Work out the finished part from the listing and answer in its coordinate system (mm). A direction names the side the tool comes from. Round coordinates to 2 decimals unless told otherwise and drop trailing zeros. Write each loop counter-clockwise with the first axis right and the second up, starting at its lowest first coordinate (ties: lowest second). Pieces come first, ordered by that corner, then holes. Notation, with made-up numbers: (-25, 48) -> (31, 48) arc R11 cw to (31, 68) -> close; hole circle Ø8 at (-13, -3). An arc over 180 degrees is marked (long way). One line per question, with ' | ' between items. Start each with the question number.
```python
from build123d import *

# Parameters (mm, degrees)
SKETCH1_R               = 23.8125
BOSS_EXTRUDE1_DEPTH     = 6.35
CUT_EXTRUDE1_DEPTH      = 53.964614985
CUT_EXTRUDE1_DEPTH_BACK = 53.964614985
SKETCH4_R               = 1.75768
BOSS_EXTRUDE3_START     = -6.35
BOSS_EXTRUDE3_DEPTH     = 6.35
SKETCH13_W              = 24.51582
SKETCH13_H              = 34.16660521
BOSS_EXTRUDE7_DEPTH     = 2.2225
SKETCH14_W              = 18.4
SKETCH14_H              = 4.571
BOSS_EXTRUDE8_DEPTH     = 12.423266239
SKETCH19_W              = 1.60782
SKETCH19_H              = 34.16660521
BOSS_EXTRUDE14_DEPTH    = 12.423266239
SKETCH20_W              = 14.645766239
SKETCH20_H              = 34.16660521
BOSS_EXTRUDE15_DEPTH    = 0.455043
CUT_EXTRUDE2_DEPTH      = 4.8895
SKETCH25_W              = 11.467193476
SKETCH25_H              = 6.35
CUT_EXTRUDE3_DEPTH      = 4.7625
SKETCH23_R              = 1.0414
CUT_EXTRUDE4_DEPTH      = 17.78
SKETCH27_R              = 1.0414
CUT_EXTRUDE5_DEPTH      = 12.7
BOSS_EXTRUDE17_START    = -34.16660521
BOSS_EXTRUDE17_DEPTH    = 34.16660521
SKETCH31_W              = 6.35
SKETCH31_H              = 8.89
CUT_EXTRUDE6_DEPTH      = 7.874


with BuildPart() as part:
    # Sketch1 → Boss-Extrude1 (new body)
    with BuildSketch(Plane(origin=(0, 0, 0), x_dir=(1, 0, 0), z_dir=(0, 1, 0))):
        with BuildLine():
            Line((-26.577499234, -4.686330195), (-36.895822467, -6.505728976))
            ThreePointArc((-36.895822467, -6.505728976), (-32.445641753, -18.7325), (-24.082037797, -28.699855061))
            Line((-24.082037797, -28.699855061), (-17.347230616, -20.673624409))
            ThreePointArc((-17.347230616, -20.673624409), (0, -26.9875), (17.347230616, -20.673624409))
            Line((17.347230616, -20.673624409), (24.082037797, -28.699855061))
            ThreePointArc((24.082037797, -28.699855061), (32.445641753, -18.7325), (36.895822467, -6.505728976))
            Line((36.895822467, -6.505728976), (26.577499234, -4.686330195))
            ThreePointArc((26.577499234, -4.686330195), (23.371860585, 13.49375), (9.230268618, 25.359954603))
            Line((9.230268618, 25.359954603), (12.81378467, 35.205584038))
            ThreePointArc((12.81378467, 35.205584038), (0, 37.465), (-12.81378467, 35.205584038))
            Line((-12.81378467, 35.205584038), (-9.230268618, 25.359954603))
            ThreePointArc((-9.230268618, 25.359954603), (-22.106865795, 15.479394076), (-26.9875, 0))
            ThreePointArc((-26.9875, 0), (-26.884804415, -2.352115607), (-26.577499234, -4.686330195))
        make_face()
        with BuildLine():
            ThreePointArc((20.006273745, -18.112817756), (23.371860585, -13.49375), (25.689297184, -8.269532421))
            Line((25.689297184, -8.269532421), (32.934160714, -9.546997332))
            ThreePointArc((32.934160714, -9.546997332), (29.696011096, -17.145), (24.735022577, -23.748321164))
            Line((24.735022577, -23.748321164), (20.006273745, -18.112817756))
        make_face(mode=Mode.SUBTRACT)
        with BuildLine():
            Line((-32.934160714, -9.546997332), (-25.689297184, -8.269532421))
            ThreePointArc((-25.689297184, -8.269532421), (-23.371860585, -13.49375), (-20.006273745, -18.112817756))
            Line((-20.006273745, -18.112817756), (-24.735022577, -23.748321164))
            ThreePointArc((-24.735022577, -23.748321164), (-29.696011096, -17.145), (-32.934160714, -9.546997332))
        make_face(mode=Mode.SUBTRACT)
        with Locations(Location((0, 0, 0), (0, 0, 270))):
            Circle(SKETCH1_R, mode=Mode.SUBTRACT)
        with BuildLine():
            ThreePointArc((-8.199138137, 33.295318497), (0, 34.29), (8.199138137, 33.295318497))
            Line((8.199138137, 33.295318497), (5.683023438, 26.382350177))
            ThreePointArc((5.683023438, 26.382350177), (0, 26.9875), (-5.683023438, 26.382350177))
            Line((-5.683023438, 26.382350177), (-8.199138137, 33.295318497))
        make_face(mode=Mode.SUBTRACT)
    extrude(amount=BOSS_EXTRUDE1_DEPTH)

    # Sketch4 → Cut-Extrude1 (cut, two sides: drawn at the far end of the back side and taken through both)
    with BuildSketch(Plane(origin=(0, 0, 0), x_dir=(0, 0, -1), z_dir=(1, 0, 0)).offset(-CUT_EXTRUDE1_DEPTH_BACK)):
        with Locations((0, 3.071710122)):
            Circle(SKETCH4_R)
    extrude(amount=CUT_EXTRUDE1_DEPTH + CUT_EXTRUDE1_DEPTH_BACK, mode=Mode.SUBTRACT)

    # Sketch7 → Boss-Extrude3 (add)
    with BuildSketch(Plane(origin=(0, 6.35, 0), x_dir=(1, 0, 0), z_dir=(0, 1, 0)).offset(BOSS_EXTRUDE3_START)):
        with BuildLine():
            Line((11.940053077, -31.683419289), (11.940053077, -24.202485177))
            ThreePointArc((11.940053077, -24.202485177), (0.536822134, -26.98216037), (-10.967946923, -24.658250071))
            Line((-10.967946923, -24.658250071), (-10.967946923, -31.683419289))
            Line((-10.967946923, -31.683419289), (11.940053077, -31.683419289))
        make_face()
        with BuildLine():
            ThreePointArc((-14.002916152, -19.26015305), (0, -23.8125), (14.002916152, -19.26015305))
            Line((14.002916152, -19.26015305), (-14.002916152, -19.26015305))
        make_face()
    extrude(amount=BOSS_EXTRUDE3_DEPTH)

    # Sketch13 → Boss-Extrude7 (add)
    with BuildSketch(Plane.XY.offset(31.683419289)):
        with Locations((1.289963077, -10.733302605)):
            Rectangle(SKETCH13_W, SKETCH13_H)
    extrude(amount=BOSS_EXTRUDE7_DEPTH)

    # Sketch14 → Boss-Extrude8 (add)
    with BuildSketch(Plane(origin=(0, 0, 31.683419289), x_dir=(-1, 0, 0), z_dir=(0, 0, -1))):
        with Locations((-2.740053077, -25.53110521)):
            Rectangle(SKETCH14_W, SKETCH14_H)
    extrude(amount=BOSS_EXTRUDE8_DEPTH)

    # Sketch19 → Boss-Extrude14 (add)
    with BuildSketch(Plane(origin=(0, 0, 31.683419289), x_dir=(-1, 0, 0), z_dir=(0, 0, -1))):
        with Locations((-12.743963077, -10.733302605)):
            Rectangle(SKETCH19_W, SKETCH19_H)
    extrude(amount=BOSS_EXTRUDE14_DEPTH)

    # Sketch20 → Boss-Extrude15 (add)
    with BuildSketch(Plane(origin=(13.547873077, 0, 0), x_dir=(0, 0, -1), z_dir=(1, 0, 0))):
        with Locations((-26.58303617, -10.733302605)):
            Rectangle(SKETCH20_W, SKETCH20_H)
    extrude(amount=BOSS_EXTRUDE15_DEPTH)

    # Sketch21 → Cut-Extrude2 (cut)
    with BuildSketch(Plane.XZ):
        Polygon((-6.459946923, 19.26015305), (-6.459946923, 30.299813914), (-6.459946923, 31.683419289), (-9.467946923, 31.683419289), (-9.467946923, 30.629419289), (-9.467946923, 19.26015305), align=None)
    extrude(amount=-CUT_EXTRUDE2_DEPTH, mode=Mode.SUBTRACT)

    # Sketch25 → Cut-Extrude3 (cut)
    with BuildSketch(Plane.ZY.offset(10.967946923)):
        with Locations((28.172322551, 3.175)):
            Rectangle(SKETCH25_W, SKETCH25_H)
    extrude(amount=CUT_EXTRUDE3_DEPTH, mode=Mode.SUBTRACT)

    # Sketch23 → Cut-Extrude4 (cut)
    with BuildSketch(Plane.ZY.offset(10.967946923)):
        with Locations((25.179419289, 2.28739479)):
            Circle(SKETCH23_R)
    extrude(amount=-CUT_EXTRUDE4_DEPTH, mode=Mode.SUBTRACT)

    # Sketch27 → Cut-Extrude5 (cut)
    with BuildSketch(Plane.ZY.offset(6.459946923)):
        with Locations((25.179419289, -25.21260521)):
            Circle(SKETCH27_R)
    extrude(amount=-CUT_EXTRUDE5_DEPTH, mode=Mode.SUBTRACT)

    # Sketch29 → Boss-Extrude17 (add)
    with BuildSketch(Plane(origin=(0, 6.35, 0), x_dir=(1, 0, 0), z_dir=(0, 1, 0)).offset(BOSS_EXTRUDE17_START)):
        with BuildLine():
            Line((17.347230616, -20.673624409), (14.002916152, -19.26015305))
            Line((14.002916152, -19.26015305), (14.002916152, -20.673624409))
            Line((14.002916152, -20.673624409), (14.002916152, -20.706319513))
            Line((14.002916152, -20.706319513), (14.002916152, -23.07040302))
            ThreePointArc((14.002916152, -23.07040302), (15.720816217, -21.935840392), (17.347230616, -20.673624409))
        make_face()
        with BuildLine():
            Line((17.347230616, -20.673624409), (14.002916152, -33.905919289))
            Line((14.002916152, -33.905919289), (14.002916152, -23.07040302))
            ThreePointArc((14.002916152, -23.07040302), (15.720816217, -21.935840392), (17.347230616, -20.673624409))
        make_face()
    extrude(amount=BOSS_EXTRUDE17_DEPTH)

    # Sketch31 → Cut-Extrude6 (cut)
    with BuildSketch(Plane(origin=(0, 6.35, 0), x_dir=(1, 0, 0), z_dir=(0, 1, 0))):
        with Locations((6.901888069, -25.428029678)):
            Rectangle(SKETCH31_W, SKETCH31_H)
    extrude(amount=-CUT_EXTRUDE6_DEPTH, mode=Mode.SUBTRACT)


solid = part.part
```
(1) A cutting plane is placed at B-B, the plane z = -30.5. Determine the outline of the cut face in (x, y), then the cut area to 3 significant figures.
(2) A cutting plane is placed at A-A, the plane x = 0. Count the separate pieces of the cut face and the enclosed holes in it, then the cut area to 3 significant figures.
(3) A cutting plane is placed at C-C, the plane x = 22.5. Determine the outline of the cut face in (y, z), then the cut area to 3 significant figures.
(4) Consider L1, parallel to Y at x = -24.5, z = 0; L2, parallel to Z at x = -5.5, y = 2.5; L3, parallel to Z at x = -2.5, y = -2.5. Determine where each line is inside the solid, lowest interval first.
(5) The mould has two halves that part along Z. Classify faces 1 (the flat face through (-11.047, 3.131, -30.352)), 2 (the cylindrical face through (-10.228, 2.6, 26.173)), 3 (the cylindrical face through (32.354, 3.131, 18.891)), 4 (the flat face through (1, 0, 25)): +Z half, -Z half, draft (parallel to the pull), parting line (faces both ways), or undercut.
(6) Given pin 1 Ø1.9 at (x, y) = (5.5, 3.5) entering from -Z; pin 2 Ø3.5 at (y, z) = (-13.5, 29.5) entering from -X; pin 3 Ø1.2 at (x, y) = (-12.5, 4.5) entering from +Z; pin 4 Ø18.5 at (x, y) = (-2.5, -5) entering from -Z (3 decimals), each flat-ended and moving along its own axis, determine where each tip first touches the part or whether it passes through.
(7) For faces 5 (the cylindrical face through (-23.412, 3.131, 13.424)), 6 (the cylindrical face through (-16.211, 3.131, 21.576)), 7 (the flat face through (-8, 4.89, 26)), determine the directions among +Z, -Z, +X, -X, +Y, -Y from which every point of the face is accessible in a straight line to the end or side of a thin tool.
(8) A cutting plane is placed at D-D, the plane y = -4.5. Determine the outline of the cut face in (x, z), then the cut area to 3 significant figures.
Returned:
1) outline: (-11.1, 0) -> (-7.18, 0) -> (-7.18, 6.35) -> (-11.1, 6.35) -> close; (7.18, 0) -> (11.1, 0) -> (11.1, 6.35) -> (7.18, 6.35) -> close | area: 49.8 mm2
2) separate pieces: 3 | enclosed holes: 2 | area: 245 mm2
3) outline: (0, -14.9) -> (6.35, -14.9) -> (6.35, -7.8) -> (0, -7.8) -> close; (0, 7.8) -> (6.35, 7.8) -> (6.35, 14.9) -> (0, 14.9) -> close; (0, 21.08) -> (6.35, 21.08) -> (6.35, 26.81) -> (0, 26.81) -> close | area: 127 mm2
4) L1: 0 to 1.31, 4.83 to 6.35 | L2: -37.06 to -33.85, -26.42 to -23.17, 19.26 to 24.16, 26.2 to 33.91 | L3: 31.68 to 33.91
5) face 1: undercut | face 2: undercut | face 3: +Z half | face 4: draft
6) pin 1: z = -37.19 | pin 2: x = 11.94 | pin 3: z = 22.44 | pin 4: z = -37.465
7) face 5: +Y, -Y | face 6: +Z, +Y, -Y | face 7: -Y
8) outline: (-10.97, 31.68) -> (11.94, 31.68) -> (11.94, 19.26) -> (14, 19.26) -> (17.35, 20.67) -> (14, 33.91) -> (-10.97, 33.91) -> close | area: 106 mm2
